Check sheet for the drawn part. Datum: minimum x, y, z corner. Units: mm. A direction names the side the tool comes from. Round coordinates to 2 decimals unless told otherwise and drop trailing zeros. Write each loop counter-clockwise with the first axis right and the second up, starting at its lowest first coordinate (ties: lowest second). Pieces come first, ordered by that corner, then holes. Notation, with made-up numbers: M -22,-31.5 L 29,-31.5 A20 cw 29,-15.5 Z; hole C -22,62.25 d5. An arc over 180 degrees is marked long. One line per item, written item: value. Start each with the question number.
1. Scan lines: probe 1 along X at (y, z) = (62, 64.5) (1 decimal); probe 2 along Z at (x, y) = (47, 32.5). Record each from-to range of solid material in increasing order. Write a range as [from, to].
2. Depth check by flat-ended pin: P1, Ø12, axis at x = 127.5, y = 12, coming from the +Z side; P2, Ø22.5, axis at x = 199.5, y = 31.5, coming from the +Z side. Enter the tip coordinate at first touch or a pass-through.
3. Release check for a two-part mould opening along X. For the marked faces 1, 2, 3 and 4 record: pulls with the +X half, pulls with the -X half, needs draft (parallel to the pull), parting line crosses it, or undercut.
4. Section check B-B (z = 71). Record the boundary of the cut face in (x, y) (1 decimal), and give its area (3 significant figures).
5. Section check C-C (y = 14.5). Record the boundary of the cut face in (x, z) (1 decimal), and give its area (3 significant figures).
6. Section check A-A (z = 89.5). Record the boundary of the cut face in (x, y) (1 decimal).
7. Access from +Z, -Z, +X, -X, +Y, -Y to the whole of each face (thin tool, end or side, straight path). Record for the marked faces 5, 6 and 7.
8. Section check D-D (x = 191). Record the boundary of the cut face in (y, z) (1 decimal), and give its area (3 significant figures).
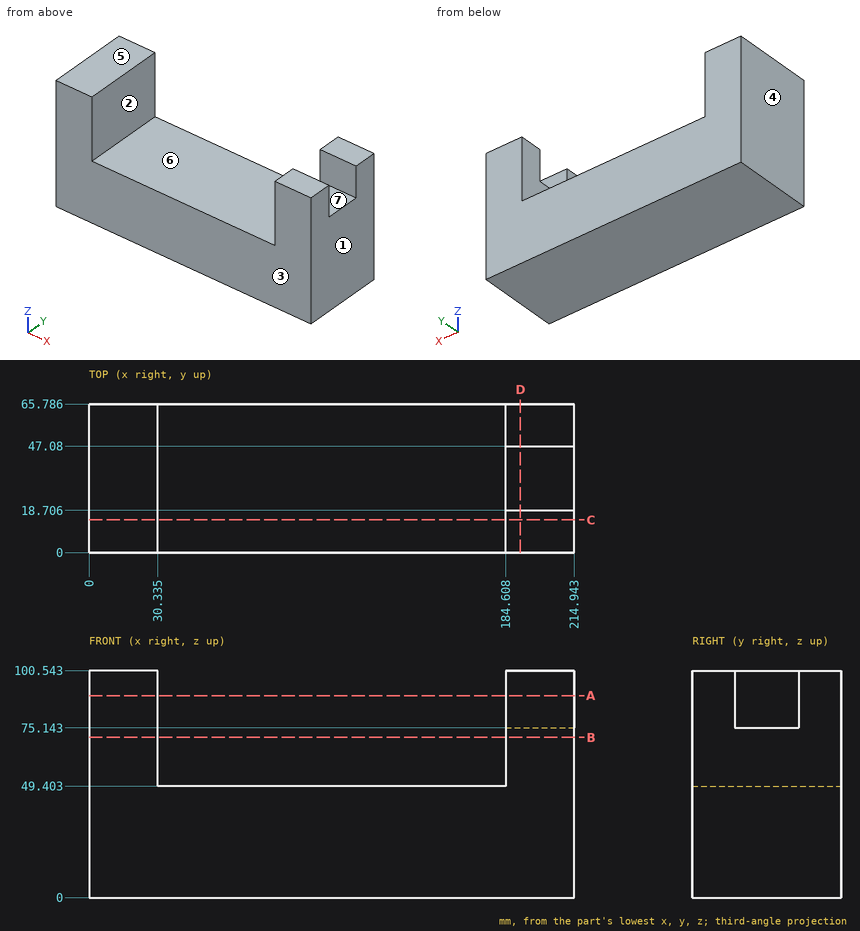
Result sheet:
1. probe 1: x = [0, 30.3], [184.6, 214.9]
1. probe 2: z = [0, 49.4]
2. P1: stops at z = 49.4
2. P2: stops at z = 75.14
3. face 1: pulls with the +X half
3. face 2: undercut
3. face 3: needs draft
3. face 4: pulls with the -X half
4. outline: M 0,0 L 30.3,0 L 30.3,65.8 L 0,65.8 Z; M 184.6,0 L 214.9,0 L 214.9,65.8 L 184.6,65.8 Z
4. area: 3,990 mm2
5. outline: M 0,0 L 214.9,0 L 214.9,100.5 L 184.6,100.5 L 184.6,49.4 L 30.3,49.4 L 30.3,100.5 L 0,100.5 Z
5. area: 13,700 mm2
6. outline: M 0,0 L 30.3,0 L 30.3,65.8 L 0,65.8 Z; M 184.6,0 L 214.9,0 L 214.9,18.7 L 184.6,18.7 Z; M 184.6,47.1 L 214.9,47.1 L 214.9,65.8 L 184.6,65.8 Z
7. face 5: +Z, +X, -X, +Y, -Y
7. face 6: +Z, +Y, -Y
7. face 7: +Z, +X
8. outline: M 0,0 L 65.8,0 L 65.8,100.5 L 47.1,100.5 L 47.1,75.1 L 18.7,75.1 L 18.7,100.5 L 0,100.5 Z
8. area: 5,890 mm2
